Source: CAD feature listing. Evaluate the final solid. Frame: model axes, mm. Face numbers are marked on the shaded views. A direction names the side the tool comes from. Give positions to 0.01 mm unless a question says otherwise; leave off trailing zeros. Loops run counter-clockwise (first coordinate to the right, second up) from the corner with the lowest first, then second, coordinate; pieces in that order, holes last. Notation, with made-up numbers: M 66,32.25 L 96,32.25 A23 ccw 96,65.25 Z; hole C -35.5,41.25 d4. An arc over 180 degrees is marked long. Put each result on its own line as item: value.
from build123d import *
from build123d.topology import SkipClean

# Parameters (mm, degrees)
SKETCH1_R           = 5
BOSS_EXTRUDE1_DEPTH = 220
CUT_EXTRUDE1_DEPTH  = 190
SKETCH4_R           = 10
CUT_EXTRUDE2_DEPTH  = 190
SKETCH5_R           = 12.5
SKETCH5_R_2         = 10
BOSS_EXTRUDE2_DEPTH = 30


with BuildPart() as part:
    # Sketch1 → Boss-Extrude1 (new, symmetric)
    with BuildSketch(Plane.XY):
        with BuildLine():
            Line((-170, 140), (170, 140))
            Line((170, 140), (170, -100))
            ThreePointArc((170, -100), (0, -160), (-170, -100))
            Line((-170, -100), (-170, 140))
        make_face()
        Circle(SKETCH1_R, mode=Mode.SUBTRACT)
    extrude(amount=BOSS_EXTRUDE1_DEPTH, both=True)

    # Sketch3 → Cut-Extrude1 (cut, symmetric)
    with BuildSketch(Plane.XY):
        with BuildLine():
            Line((-150, 140), (150, 140))
            Line((150, 140), (150, -90.207361828))
            ThreePointArc((150, -90.207361828), (116.45426588, -111.328240908), (80, -126.900469714))
            Line((80, -126.900469714), (80, -159.889880276))
            ThreePointArc((80, -159.889880276), (0, -171.462714083), (-80, -159.889880276))
            Line((-80, -159.889880276), (-80, -126.900469714))
            ThreePointArc((-80, -126.900469714), (-116.45426588, -111.328240908), (-150, -90.207361828))
            Line((-150, -90.207361828), (-150, 140))
        make_face()
    extrude(amount=CUT_EXTRUDE1_DEPTH, both=True, mode=Mode.SUBTRACT)

    # Sketch4 → Cut-Extrude2 (cut, symmetric)
    with BuildSketch(Plane.ZY.offset(-150)):
        with Locations(Location((0, 85, 0), (0, 0, 270))):
            Circle(SKETCH4_R)
    extrude(amount=CUT_EXTRUDE2_DEPTH, both=True, mode=Mode.SUBTRACT)

    # Sketch5 → Boss-Extrude2 (add)
    with SkipClean():  # the faces are left unmerged after this step: merging them gives an invalid solid
        with BuildSketch(Plane(origin=(170, 0, 0), x_dir=(0, 0, -1), z_dir=(1, 0, 0))):
            with Locations(Location((0, 85, 0), (0, 0, 270))):
                Circle(SKETCH5_R)
            with Locations(Location((0, 85, 0), (0, 0, 90))):
                Circle(SKETCH5_R_2, mode=Mode.SUBTRACT)
        extrude(amount=BOSS_EXTRUDE2_DEPTH)


solid = part.part
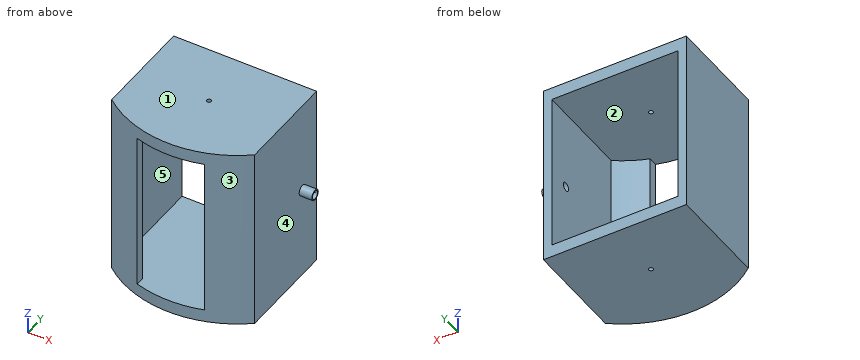
1. Access query for the marked faces 1 and 2. Directions: +Z, -Z, +X, -X, +Y, -Y. A direction counts if a zero-diameter tool reaches every point of the face in a straight line with its end or side. Return the directions, or none.
Found:
face 1: +Z, +X, -X, +Y, -Y
face 2: +Y
2. Contact query for flat-ended pins moving along their axis: P1, Ø16, axis at x = 0, y = 0, coming from the -Z side; P2, Ø10.5, axis at y = -142.5, z = 43, coming from the +X side; P3, Ø8, axis at y = 103, z = -149.5, coming from the +X side; P4, Ø17, axis at y = -140, z = -36, coming from the -X side. Output: stop coordinate, or through.
Found:
P1: z = -220
P2: x = 108.65
P3: x = 170
P4: x = -120.93
3. Section query D-D (y = 108). Output: boundary loops of the cut face in (x, z).
Found:
outline: M -170,-220 L 170,-220 L 170,220 L -170,220 Z; hole M -150,-190 L 150,-190 L 150,190 L -150,190 Z
4. Draft query along X for the marked faces 3, 4 and 5. Return one class per face: pulls with the +X half, pulls with the -X half, needs draft (parallel to the pull), parting line crosses it, or undercut.
Found:
face 3: parting line crosses it
face 4: pulls with the +X half
face 5: undercut
5. Section query C-C (z = -162). Output: boundary loops of the cut face in (x, y).
Found:
outline: M -170,-100 A270.83 ccw -80,-147.91 L -80,-126.9 A250.83 cw -150,-90.21 L -150,140 L -170,140 Z; M 80,-147.91 A270.83 ccw 170,-100 L 170,140 L 150,140 L 150,-90.21 A250.83 cw 80,-126.9 Z
6. Section query B-B (x = -18.5). Output: boundary loops of the cut face in (y, z), plus the area to 3 significant figures.
Found:
outline: M -159.37,-220 L 140,-220 L 140,-190 L -159.37,-190 Z; M -159.37,190 L 140,190 L 140,220 L -159.37,220 Z
area: 18,000 mm^2
7. Material intervals for line 1 (X direction, y = -80, z = 164); line 2 (Y direction, x = 0, z = 200); line 3 (Z direction, x = -16.5, y = -56.5), sorted ascending. Write a range as from..to.
Found:
line 1: -170..-150, 150..170
line 2: -160..-5, 5..140
line 3: -220..-190, 190..220
